from build123d import *

# Parameters (mm, degrees)
F0_W     = 38.1
F0_H     = 31.75
F1_DEPTH = 25.4
F3_DEPTH = 25.4
F6_W     = 29.6103259988
F6_H     = 31.75
F7_DEPTH = 25.4


# Not quite as in the source:
# - a feature of the source that left no trace in its solid (it failed there, or was rolled back) is left out


with BuildPart() as f1:
    # F0 (on Front) → F1 (new body)
    with BuildSketch(Plane.XZ):
        with Locations((-10.5603259988, 15.875)):
            Rectangle(F0_W, F0_H)
    extrude(amount=F1_DEPTH)

    # F2 (on face) → F3 (join)
    with BuildSketch(Plane.YZ.offset(8.4896740012)):
        Polygon((-6.35, 31.75), (-25.4, 6.35), (-25.4, 0), (0, 0), (0, 31.75), align=None)
    extrude(amount=F3_DEPTH)

    # F6 (on face) → F7 (cut)
    with BuildSketch(Plane.XZ.offset(25.4)):
        with Locations((-14.8051629994, 15.875)):
            Rectangle(F6_W, F6_H)
    extrude(amount=-F7_DEPTH, mode=Mode.SUBTRACT)


solid = f1.part
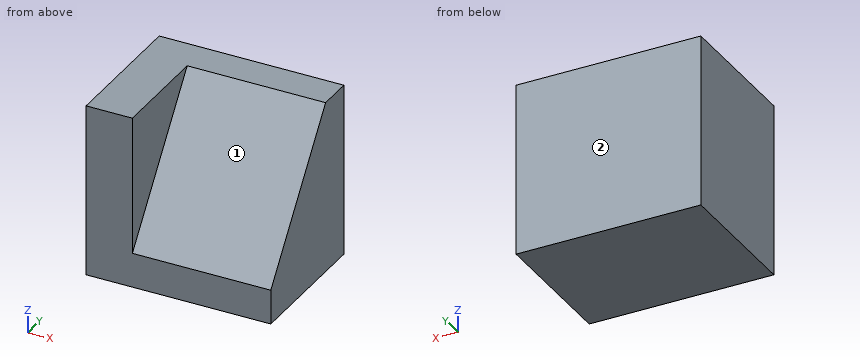
Read the model definition and answer for the solid it produces. Units are mm, in the model's axes. Face numbers are marked on the shaded views. A direction names the side the tool comes from. Give positions to 0.01 mm unless a question says otherwise; leave off trailing zeros. Write each loop counter-clockwise with the first axis right and the second up, starting at its lowest first coordinate (ties: lowest second). Pieces come first, ordered by that corner, then holes. Notation, with made-up numbers: (74, -5.75) -> (92, -5.75) arc R8 ccw to (92, 9.25) -> close; hole circle Ø11 at (-26.5, 62.25). An arc over 180 degrees is marked (long way). Answer as a JSON object with one key per item and string values. Group by question number.
1) Each of these flat-tipped pins is pushed along its axis until it touches: P1, Ø6, axis at x = 13.5, y = -12.5, coming from the +Z side; P2, Ø8, axis at x = 27, y = -10.5, coming from the +Z side. Where does it stop, or does it pass through?
2) A tool of negligible diameter and unlimited length cuts with its end or side. For the marked faces 1 and 2, from which of +Z, -Z, +X, -X, +Y, -Y can it reach the whole face along a straight path? Write none if from no direction.
3) Find section C-C (z = 29). Write down the section's boundary in (x, y).
4) Find section B-B (x = 10). Write down the section's boundary in (y, z).
5) Consider L1, parallel to X at y = -17.5, z = 27; L2, parallel to Y at x = 31, z = 22; L3, parallel to Z at x = 23.5, y = -16.5. Determine where each line is inside the solid, lowest interval first. Write a range as from..to.
6) Find section A-A (y = -8). Write down the section's boundary in (x, z), and give its area (3 significant figures).
Values follow:
{
 "1": {"P1": "stops at z = 27.55", "P2": "stops at z = 31.55"},
 "2": {"face 1": "+Z, +X, -Y", "face 2": "+Z, -Z, +X, -X, +Y"},
 "3": {"outline": "(0, -25.4) -> (8.49, -25.4) -> (8.49, -8.41) -> (33.89, -8.41) -> (33.89, 0) -> (0, 0) -> close"},
 "4": {"outline": "(-25.4, 0) -> (0, 0) -> (0, 31.75) -> (-6.35, 31.75) -> (-25.4, 6.35) -> close"},
 "5": {"L1": "x = 0..8.49", "L2": "y = -13.66..0", "L3": "z = 0..18.22"},
 "6": {"outline": "(0, 0) -> (33.89, 0) -> (33.89, 29.55) -> (8.49, 29.55) -> (8.49, 31.75) -> (0, 31.75) -> close", "area": "1,020 mm2"}
}
